from build123d import *

# Parameters (mm, degrees)
CROQUIS1_R              = 9
SALIENTE_EXTRUIR1_DEPTH = 60
CROQUIS3_W              = 46
CROQUIS3_H              = 7
CORTAR_EXTRUIR1_DEPTH   = 36
CROQUIS4_W              = 47.607342582
CROQUIS4_H              = 24
CORTAR_EXTRUIR5_DEPTH   = 36


with BuildPart() as part:
    # Croquis1 → Saliente-Extruir1 (new body)
    with BuildSketch(Plane.XY):
        Polygon((-23, 0), (23, 0), (23, 32), (12.720887074, 48), (-11.279112926, 48), (-23, 32), align=None)
        with Locations((0, 32)):
            Circle(CROQUIS1_R, mode=Mode.SUBTRACT)
    extrude(amount=-SALIENTE_EXTRUIR1_DEPTH)

    # Croquis3 → Cortar-Extruir1 (cut)
    with BuildSketch(Plane(origin=(0, 48, 0), x_dir=(1, 0, 0), z_dir=(0, 1, 0))):
        with Locations((0, 3.5)):
            Rectangle(CROQUIS3_W, CROQUIS3_H)
        with Locations((0, 56.5)):
            Rectangle(CROQUIS3_W, CROQUIS3_H)
    extrude(amount=-CORTAR_EXTRUIR1_DEPTH, mode=Mode.SUBTRACT)

    # Croquis4 → Cortar-Extruir5 (cut)
    with BuildSketch(Plane(origin=(0, 48, 0), x_dir=(1, 0, 0), z_dir=(0, 1, 0))):
        with Locations((0.803671291, 30)):
            Rectangle(CROQUIS4_W, CROQUIS4_H)
    extrude(amount=-CORTAR_EXTRUIR5_DEPTH, mode=Mode.SUBTRACT)


solid = part.part
Model file for the job. Use its own axes, mm. A direction names the side the tool comes from. Round coordinates to 2 decimals unless told otherwise and drop trailing zeros. Order: outer loops, then holes, each group sorted by start corner. A loop starts at its lowest first (then second) coordinate and runs counter-clockwise, first axis right, second up.
(1) Drill centre lines: line 1 (Y direction, x = 0, z = -13); line 2 (Z direction, x = -8.5, y = 15); line 3 (Y direction, x = -6, z = -24). Where is each one in solid material? Low to high.
(2) Band-saw the part on D-D (x = -14). List the corners of the cut face in (y, z), then the cut area to 3 significant figures.
(3) Pin check, flat tips, straight feed: pin 1 (4 mm diameter, centred on y = 39, z = -45.5, fed in from -X); pin 2 (3 mm diameter, centred on x = 9.5, z = -24, fed in from +Y); pin 3 (11 mm diameter, centred on x = -7, y = 27.5, fed in from +Z). Stop position of each tip, or through.
(4) 3-axis set-ups, long thin cutter, end or side, ignore diameter. For faces 1 (the face through (-17.06, 40.11, -47.42)), 2 (the face through (0, 12, -4)), 3 (the face through (0, 22, -42)), 4 (the face through (0, 6, 0)), 5 (the face through (0, 12, -57)): which of +Z, -Z, +X, -X, +Y, -Y reach the whole face in a straight line?
(5) Pull direction Z, two halves, no side cores. Call faces 6 (the face through (17.93, 39.89, -12.42)), 7 (the face through (0, 22, -18)), 8 (the face through (0, 22, -53)): released by +Z, released by -Z, zero draft, split by the parting line, or undercut.
(6) Band-saw the part on A-A (x = 0). List the corners of the cut face in (y, z).
(7) Band-saw the part on B-B (y = 42.5). List the corners of the cut face in (x, z).
(8) Band-saw the part on C-C (z = -14.5). List the corners of the cut face in (x, y), then the cut area to 3 significant figures.
Verdict:
1. line 1: y = 0 to 23, 41 to 48
1. line 2: z = -53 to -42, -18 to -7
1. line 3: y = 0 to 12
2. outline: (0, -60) - (12, -60) - (12, -53) - (44.29, -53) - (44.29, -42) - (12, -42) - (12, -18) - (44.29, -18) - (44.29, -7) - (12, -7) - (12, 0) - (0, 0) - close
2. area: 1,430 mm2
3. pin 1: stops at x = -19.34
3. pin 2: stops at y = 12
3. pin 3: stops at z = -7
4. face 1: +Z, -Z, -X, +Y
4. face 2: +Z, +X, -X, +Y
4. face 3: +X, -X, +Y
4. face 4: +Z, +X, -X, +Y, -Y
4. face 5: -Z, +X, -X, +Y
5. face 6: zero draft
5. face 7: undercut
5. face 8: released by -Z
6. outline: (0, -60) - (12, -60) - (12, -53) - (23, -53) - (23, -42) - (12, -42) - (12, -18) - (23, -18) - (23, -7) - (12, -7) - (12, 0) - (0, 0) - close; (41, -53) - (48, -53) - (48, -42) - (41, -42) - close; (41, -18) - (48, -18) - (48, -7) - (41, -7) - close
7. outline: (-15.31, -53) - (16.25, -53) - (16.25, -42) - (-15.31, -42) - close; (-15.31, -18) - (16.25, -18) - (16.25, -7) - (-15.31, -7) - close
8. outline: (-23, 0) - (23, 0) - (23, 32) - (12.72, 48) - (-11.28, 48) - (-23, 32) - close; hole circle Ø18 at (0, 32)
8. area: 1,780 mm2
